The listing builds one solid part. Answer for the finished solid, in the listing's coordinates (mm). A direction names the side the tool comes from. Round coordinates to 2 decimals unless told otherwise and drop trailing zeros. Loops run counter-clockwise (first coordinate to the right, second up) from the corner with the lowest first, then second, coordinate; pieces in that order, holes last. Notation, with made-up numbers: (70.5, -12.5) -> (75.5, -12.5) arc R19 cw to (75.5, 19.5) -> close; hole circle Ø5 at (28.25, -35.75). An arc over 180 degrees is marked (long way). One line per question, with ' | ' between items.
from build123d import *

# Parameters (mm, degrees)
SKETCH1_W           = 120
SKETCH1_H           = 100
BOSS_EXTRUDE1_DEPTH = 40
BOSS_EXTRUDE2_DEPTH = 120
CUT_EXTRUDE2_DEPTH  = 1


with BuildPart() as part:
    # Sketch1 → Boss-Extrude1 (new body)
    with BuildSketch(Plane(origin=(0, 0, 0), x_dir=(1, 0, 0), z_dir=(0, 1, 0))):
        Rectangle(SKETCH1_W, SKETCH1_H)
    extrude(amount=BOSS_EXTRUDE1_DEPTH)

    # Sketch2 → Boss-Extrude2 (add)
    with BuildSketch(Plane(origin=(60, 0, 0), x_dir=(0, 0, -1), z_dir=(1, 0, 0))):
        Polygon((-3.8, 40), (-6.20177712, 44.16), (6.20177712, 44.16), (3.8, 40), align=None)
    extrude(amount=-BOSS_EXTRUDE2_DEPTH)

    # Sketch5 → Cut-Extrude2 (cut)
    with BuildSketch(Plane.XZ):
        Polygon((-10.888743303, -30.135074667), (-10.888743303, 13.324383252), (-25.483702069, 13.324383252), (0, 40.546241509), (25.483702069, 13.324383252), (10.888743303, 13.324383252), (10.888743303, -30.135074667), align=None)
    extrude(amount=-CUT_EXTRUDE2_DEPTH, mode=Mode.SUBTRACT)


solid = part.part
Q1. A cutting plane is placed at A-A on z = -25. Give the vertices of the cut face in (x, y).
Numbers:
outline: (-60, 0) -> (-10.89, 0) -> (-10.89, 1) -> (10.89, 1) -> (10.89, 0) -> (60, 0) -> (60, 40) -> (-60, 40) -> close
Q2. A cutting plane is placed at D-D on x = -20.5. Give the vertices of the cut face in (y, z), plus the area to 3 significant figures.
Numbers:
outline: (0, -50) -> (40, -50) -> (40, -3.8) -> (44.16, -6.2) -> (44.16, 6.2) -> (40, 3.8) -> (40, 50) -> (0, 50) -> (0, 18.65) -> (1, 18.65) -> (1, 13.32) -> (0, 13.32) -> close | area: 4,040 mm^2
Q3. For faces 5 (the face through (-60, 22, 1)), 6 (the face through (12.56, 0.49, 27.13)), determine the directions among +Z, -Z, +X, -X, +Y, -Y from which every point of the face is accessible in a straight line to the end or side of a thin tool.
Numbers:
face 5: +Z, -Z, -X, +Y, -Y | face 6: -Y
Q4. Find the intervals of material crossed by line 1 (Y direction, x = -51.5, z = 45.5); line 2 (Y direction, x = -16, z = -5.5); line 3 (Y direction, x = -8, z = 12.5), in increasing order. Write a range as from..to.
Numbers:
line 1: 0..40 | line 2: 0..40, 42.94..44.16 | line 3: 1..40
Q5. Given pin 1 Ø12 at (x, z) = (-46, 37) entering from -Y; pin 2 Ø23 at (x, z) = (23.5, -36) entering from +Y; pin 3 Ø5 at (x, z) = (-5, 11.5) entering from -Y, each flat-ended and moving along its own axis, determine where each tip first touches the part or whether it passes through.
Numbers:
pin 1: y = 0 | pin 2: y = 40 | pin 3: y = 1
Q6. A cutting plane is placed at B-B on x = 46.5. Give the vertices of the cut face in (y, z).
Numbers:
outline: (0, -50) -> (40, -50) -> (40, -3.8) -> (44.16, -6.2) -> (44.16, 6.2) -> (40, 3.8) -> (40, 50) -> (0, 50) -> close
Q7. For a pull along Y with two mould halves and no side action, classify faces 1 (the face through (0.84, 42.051, 4.984)), 2 (the face through (-1, 20, -50)), 3 (the face through (0.84, 42.11, -5.02)), 4 (the face through (-14, 0, -1)) as pulls with the +Y half, pulls with the -Y half, needs draft (parallel to the pull), parting line crosses it, or undercut.
Numbers:
face 1: undercut | face 2: needs draft | face 3: undercut | face 4: pulls with the -Y half
Q8. A cutting plane is placed at C-C on z = -42. Give the vertices of the cut face in (x, y), plus the area to 3 significant figures.
Numbers:
outline: (-60, 0) -> (60, 0) -> (60, 40) -> (-60, 40) -> close | area: 4,800 mm^2
